```python
from build123d import *

# Parameters (mm, degrees)
SKETCH1_R               = 34.925
BOSS_EXTRUDE1_DEPTH     = 19.05
SKETCH2_W               = 106.68
SKETCH2_H               = 26.67
CUT_EXTRUDE1_DEPTH      = 19.05
SKETCH4_W               = 76.2
SKETCH4_H               = 35.56
CUT_EXTRUDE2_DEPTH      = 10
SKETCH5_R               = 17.78
CUT_EXTRUDE3_DEPTH      = 10
CUT_EXTRUDE4_DEPTH      = 53.937829102
CUT_EXTRUDE4_DEPTH_BACK = 53.937829102
SKETCH6_R               = 3.175
CUT_EXTRUDE5_DEPTH      = 53.937829102
CUT_EXTRUDE5_DEPTH_BACK = 53.937829102
SKETCH7_W               = 12.7
SKETCH7_H               = 106.569119896


with BuildPart() as part:
    # Sketch1 → Boss-Extrude1 (new body)
    with BuildSketch(Plane.XY):
        with Locations(Location((0, 0, 0), (0, 0, 180))):
            Circle(SKETCH1_R)
    extrude(amount=BOSS_EXTRUDE1_DEPTH)

    # Sketch2 → Cut-Extrude1 (cut)
    with BuildSketch(Plane.XY.offset(19.05)):
        with Locations((-34.925, 0)):
            Rectangle(SKETCH2_W, SKETCH2_H)
    extrude(amount=-CUT_EXTRUDE1_DEPTH, mode=Mode.SUBTRACT)

    # Sketch4 → Cut-Extrude2 (cut)
    with BuildSketch(Plane.XY.offset(19.05)):
        with Locations((-38.1, 0)):
            Rectangle(SKETCH4_W, SKETCH4_H)
    extrude(amount=-CUT_EXTRUDE2_DEPTH, mode=Mode.SUBTRACT)

    # Sketch5 → Cut-Extrude3 (cut)
    with BuildSketch(Plane.XY.offset(19.05)):
        Circle(SKETCH5_R)
    extrude(amount=-CUT_EXTRUDE3_DEPTH, mode=Mode.SUBTRACT)

    # Sketch6 → Cut-Extrude4 (cut, two sides: drawn at the far end of the back side and taken through both)
    with BuildSketch(Plane.XY.offset(19.05).offset(-CUT_EXTRUDE4_DEPTH_BACK)):
        with Locations((0, 27.94)):
            Circle(SKETCH6_R)
        with Locations((0, -27.94)):
            Circle(SKETCH6_R)
    extrude(amount=CUT_EXTRUDE4_DEPTH + CUT_EXTRUDE4_DEPTH_BACK, mode=Mode.SUBTRACT)

    # Sketch7 → Cut-Extrude5 (cut, two sides: drawn at the far end of the back side and taken through both)
    with BuildSketch(Plane.XY.offset(19.05).offset(-CUT_EXTRUDE5_DEPTH_BACK)):
        with Locations((34.925, 0)):
            Rectangle(SKETCH7_W, SKETCH7_H)
    extrude(amount=CUT_EXTRUDE5_DEPTH + CUT_EXTRUDE5_DEPTH_BACK, mode=Mode.SUBTRACT)


solid = part.part
```
For this review, take the finished solid that the model builds, in its own axes (mm). A direction names the side the tool comes from. Round coordinates to 2 decimals unless told otherwise and drop trailing zeros. Write each loop counter-clockwise with the first axis right and the second up, starting at its lowest first coordinate (ties: lowest second). Pieces come first, ordered by that corner, then holes. Notation, with made-up numbers: (-40, 44.25) -> (8, 44.25) arc R31 cw to (8, 69.25) -> close; hole circle Ø11 at (76.25, 63). An arc over 180 degrees is marked (long way). Use one line per item in the form item = value.
Q1. To check wall thickness, follow probe 1 along Y at (x, z) = (0, 11.25) (3 decimals); probe 2 along Y at (x, z) = (0, 7.75) (3 decimals); probe 3 along Y at (x, z) = (4, 5.5) (3 decimals). State the ranges of each line that lie inside material, in increasing order. Write a range as from..to.
Resolved:
probe_1 = -34.925..-31.115, -24.765..-17.78, 17.78..24.765, 31.115..34.925
probe_2 = -34.925..-31.115, -24.765..-13.335, 13.335..24.765, 31.115..34.925
probe_3 = -34.695..-13.335, 13.335..34.695
Q2. Machinability: for faces 5 (the flat face through (18.415, 0, 10)), 6 (the flat face through (19, 0, 19.05)), 7 (the flat face through (-11, -16, 9.05)), which of the approach directions +Z, -Z, +X, -X, +Y, -Y give a long, thin tool a straight path to every point of the face, cutting with its end or side? Answer none if there is none.
Resolved:
face_5 = +Z, -Z, -X
face_6 = +Z, +X, -X, +Y, -Y
face_7 = +Z, -X
Q3. Consider section A-A (z = 13.75). State the section outline as (x, y) points (3 decimals).
Resolved:
outline = (-30.06, -17.78) arc R34.925 ccw to (28.575, -20.08) -> (28.575, 20.08) arc R34.925 ccw to (-30.06, 17.78) -> (0, 17.78) arc R17.78 cw to (11.76, 13.335) -> (18.415, 13.335) -> (18.415, -13.335) -> (11.76, -13.335) arc R17.78 cw to (0, -17.78) -> close; hole circle Ø6.35 at (0, -27.94); hole circle Ø6.35 at (0, 27.94)
Q4. Consider section C-C (y = -27.94). State the section outline as (x, z) points (3 decimals).
Resolved:
outline = (-20.955, 0) -> (-3.175, 0) -> (-3.175, 19.05) -> (-20.955, 19.05) -> close; (3.175, 0) -> (20.955, 0) -> (20.955, 19.05) -> (3.175, 19.05) -> close
Q5. Consider section B-B (x = 7). State the section outline as (y, z) points (3 decimals).
Resolved:
outline = (-34.216, 0) -> (-13.335, 0) -> (-13.335, 9.05) -> (-16.344, 9.05) -> (-16.344, 19.05) -> (-34.216, 19.05) -> close; (13.335, 0) -> (34.216, 0) -> (34.216, 19.05) -> (16.344, 19.05) -> (16.344, 9.05) -> (13.335, 9.05) -> close
Q6. The part is to be moulded in two halves that separate along Y. For faces 1 (the cylindrical face through (-4.37, -34.65, 9.39)), 2 (the flat face through (28.575, 0, 9)), 3 (the cylindrical face through (-3.328, 34.766, 9.392)), 4 (the cylindrical face through (6.37, 16.6, 14.12)), say which applies: released by +Y, released by -Y, zero draft, split by the parting line, or undercut.
Resolved:
face_1 = released by -Y
face_2 = zero draft
face_3 = released by +Y
face_4 = undercut
Q7. Clearance check with flat-ended pins moving along their axes: pin 1 Ø5 at (x, z) = (-12, 13.5) entering from +Y; pin 2 Ø5 at (x, z) = (-15.5, 16.5) entering from +Y; pin 3 Ø1 at (x, z) = (6.5, 4) entering from -Y; pin 4 Ø3 at (x, y) = (14, 26) entering from -Z. State where each tip first meets the part, or that it passes through.
Resolved:
pin_1 = 33.61
pin_2 = 32.42
pin_3 = -34.41
pin_4 = 0
Q8. Consider section D-D (z = 2). State the section outline as (x, y) points (3 decimals).
Resolved:
outline = (-32.279, -13.335) arc R34.925 ccw to (28.575, -20.08) -> (28.575, 20.08) arc R34.925 ccw to (-32.279, 13.335) -> (18.415, 13.335) -> (18.415, -13.335) -> close; hole circle Ø6.35 at (0, -27.94); hole circle Ø6.35 at (0, 27.94)
